Check sheet for the modelled part. Datum: model origin and axes. Units: mm. A direction names the side the tool comes from. Coordinates: 2 decimals unless noted, no trailing zeros. Write each loop counter-clockwise with the first axis right and the second up, starting at its lowest first coordinate (ties: lowest second). Pieces come first, ordered by that corner, then holes. Notation, with made-up numbers: (60.5, -1) -> (102.5, -1) arc R16 cw to (102.5, 15) -> close; hole circle Ø10 at (-39, -33). An arc over 180 degrees is marked (long way). One line per item, written item: value. Start each with the question number.
1) Draft check along Y on faces 1 (the flat face through (26, -22, 14)), 2 (the flat face through (-3.61, -1.36, 1.73)). Enter one of: +Y half, -Y half, draft (parallel to the pull), parting line (faces both ways), or undercut.
2) Gauge pin test, flat ends, axial feed: P1, Ø3, axis at x = -5.5, y = -0.5, coming from the -Z side; P2, Ø2.5, axis at x = -1, z = 9, coming from the -Y side; P3, Ø6, axis at x = 16, y = 30, coming from the +Z side. Record the tip position at first contact, or that the pin passes through.
3) Sectioned sample at A-A on x = 25. Enter the section's corners in (y, z), plus the area to 3 significant figures.
4) Scan lines: line 1 along Y through (x, z) = (-6, 5.5); line 2 along Y through (x, z) = (28, 9); line 3 along Y through (x, z) = (6, 10). Record each from-to range of solid material in increasing order. Write a range as [from, to].
5) Sectioned sample at D-D on z = 12.75. Give the number of separate pieces and of enclosed holes in the cut face, plus the area to 3 significant figures.
6) Set-up check for faces 3 (the flat face through (21, -32, 8)), 4 (the flat face through (-10, -1, 7)), 5 (the flat face through (8.37, -39.606, 1.726)), 6 (the cylindrical face through (-0.17, -41.3, 6.4)): record each of +Z, -Z, +X, -X, +Y, -Y from which the full face is reachable in a straight line by a thin tool's end or side.
7) Sectioned sample at B-B on y = -20. Enter the section's corners in (x, z), plus the area to 3 significant figures.
8) Sectioned sample at C-C on x = 0. Enter the section's corners in (y, z), plus the area to 3 significant figures.
```python
from build123d import *

# Parameters (mm, degrees)
PAD004_DEPTH    = 5
PAD003_DEPTH    = 5
PAD002_DEPTH    = 5
PAD001_DEPTH    = 5
SKETCH_W        = 45
SKETCH_H        = 90
PAD_DEPTH       = 14
SKETCH001_R     = 7.6
POCKET_DEPTH    = 90.001
SKETCH002_R     = 1.75
POCKET001_DEPTH = 14.001
POCKET002_DEPTH = 12
SKETCH004_R     = 2.25
POCKET003_DEPTH = 14.001
SKETCH008_R     = 4.1
POCKET005_DEPTH = 20
POCKET006_DEPTH = 3.5
POCKET007_DEPTH = 5


with BuildPart() as pad004:
    # Sketch021 → Pad004 (new body)
    with BuildSketch(Plane.XZ.offset(32.5)):
        with BuildLine():
            ThreePointArc((-7.6, 14), (0, 6.4), (7.6, 14))
            Line((7.6, 14), (5, 14))
            ThreePointArc((-5, 14), (0, 9), (5, 14))
            Line((-7.6, 14), (-5, 14))
        make_face()
    extrude(amount=PAD004_DEPTH)


with BuildPart() as pad003:
    # Sketch020 → Pad003 (new body)
    with BuildSketch(Plane.XZ.offset(-32.5)):
        with BuildLine():
            ThreePointArc((-7.6, 14), (0, 6.4), (7.6, 14))
            Line((7.6, 14), (5, 14))
            ThreePointArc((-5, 14), (0, 9), (5, 14))
            Line((-7.6, 14), (-5, 14))
        make_face()
    extrude(amount=-PAD003_DEPTH)


with BuildPart() as pad002:
    # Sketch019 → Pad002 (new body)
    with BuildSketch(Plane.XZ.offset(7.5)):
        with BuildLine():
            ThreePointArc((-7.6, 14), (0, 6.4), (7.6, 14))
            Line((7.6, 14), (5, 14))
            ThreePointArc((-5, 14), (0, 9), (5, 14))
            Line((-7.6, 14), (-5, 14))
        make_face()
    extrude(amount=-PAD002_DEPTH)


with BuildPart() as pad001:
    # Sketch018 → Pad001 (new body)
    with BuildSketch(Plane.XZ.offset(-7.5)):
        with BuildLine():
            ThreePointArc((-7.6, 14), (0, 6.4), (7.6, 14))
            Line((7.6, 14), (5, 14))
            ThreePointArc((-5, 14), (0, 9), (5, 14))
            Line((-7.6, 14), (-5, 14))
        make_face()
    extrude(amount=PAD001_DEPTH)


with BuildPart() as fusion:
    # Sketch → Pad (new body)
    with BuildSketch(Plane.XY):
        with Locations((12.5, 0)):
            Rectangle(SKETCH_W, SKETCH_H)
    extrude(amount=PAD_DEPTH)

    # Sketch001 → Pocket (cut, through all)
    with BuildSketch(Plane.XZ.offset(45)):
        with Locations((0, 14)):
            Circle(SKETCH001_R)
    extrude(amount=-POCKET_DEPTH, mode=Mode.SUBTRACT)

    # Sketch002 → Pocket001 (cut, through all)
    with BuildSketch(Plane.XY.offset(14)):
        with Locations((-6, 41)):
            Circle(SKETCH002_R)
        with Locations((-6, -41)):
            Circle(SKETCH002_R)
        with Locations((6, 41)):
            Circle(SKETCH002_R)
        with Locations((6, -41)):
            Circle(SKETCH002_R)
        with Locations((6, 0)):
            Circle(SKETCH002_R)
        with Locations((-6, 0)):
            Circle(SKETCH002_R)
        with Locations((28, 41)):
            Circle(SKETCH002_R)
        with Locations((28, 23)):
            Circle(SKETCH002_R)
        with Locations((28, -23)):
            Circle(SKETCH002_R)
        with Locations((28, -41)):
            Circle(SKETCH002_R)
    extrude(amount=-POCKET001_DEPTH, mode=Mode.SUBTRACT)

    # Sketch003 → Pocket002 (cut)
    with BuildSketch(Plane.XY.offset(14)):
        Polygon((10, 50), (10, -50), (21, -50), (21, -18), (41, -18), (41, 18), (21, 18), (21, 50), align=None)
    extrude(amount=-POCKET002_DEPTH, mode=Mode.SUBTRACT)

    # Sketch004 → Pocket003 (cut, through all)
    with BuildSketch(Plane(origin=(0, 0, 0), x_dir=(1, 0, 0), z_dir=(0, 0, -1))):
        with Locations((25, 7.5)):
            Circle(SKETCH004_R)
        with Locations((25, -7.5)):
            Circle(SKETCH004_R)
    extrude(amount=-POCKET003_DEPTH, mode=Mode.SUBTRACT)

    # Sketch008 → Pocket005 (cut)
    with BuildSketch(Plane.YZ.offset(35)):
        with Locations((-32.5, 14)):
            Circle(SKETCH008_R)
        with Locations((32.5, 14)):
            Circle(SKETCH008_R)
    extrude(amount=-POCKET005_DEPTH, mode=Mode.SUBTRACT)

    # Sketch012 → Pocket006 (cut)
    with BuildSketch(Plane(origin=(0, 0, 0), x_dir=(1, 0, 0), z_dir=(0, 0, -1))):
        Polygon((-4.412285, 2.750003), (-7.587715, 2.750003), (-9.17543, 0), (-7.587715, -2.750003), (-4.412285, -2.750003), (-2.82457, 0), align=None)
        Polygon((7.587715, 2.750003), (4.412285, 2.750003), (2.82457, 0), (4.412285, -2.750003), (7.587715, -2.750003), (9.17543, 0), align=None)
        Polygon((-4.412285, 43.750003), (-7.587715, 43.750003), (-9.17543, 41), (-7.587715, 38.249997), (-4.412285, 38.249997), (-2.82457, 41), align=None)
        Polygon((7.587715, -38.249997), (4.412285, -38.249997), (2.82457, -41), (4.412285, -43.750003), (7.587715, -43.750003), (9.17543, -41), align=None)
        Polygon((7.587715, 43.750003), (4.412285, 43.750003), (2.82457, 41), (4.412285, 38.249997), (7.587715, 38.249997), (9.17543, 41), align=None)
        Polygon((-4.412285, -38.249997), (-7.587715, -38.249997), (-9.17543, -41), (-7.587715, -43.750003), (-4.412285, -43.750003), (-2.82457, -41), align=None)
    extrude(amount=-POCKET006_DEPTH, mode=Mode.SUBTRACT)

    # Sketch022 → Pocket007 (cut)
    with BuildSketch(Plane.XY.offset(2)):
        Polygon((44.573685, 18), (36, 3.425), (36, -3.425), (44.573685, -18), (55.573685, -18), (55.573685, 18), align=None)
    extrude(amount=-POCKET007_DEPTH, mode=Mode.SUBTRACT)

    # Fusion: union Pad004, Pad003, Pad002, Pad001
    add(pad004.part)
    add(pad003.part)
    add(pad002.part)
    add(pad001.part)


solid = fusion.part
```
Answers:
1. face 1: draft
1. face 2: undercut
2. P1: stops at z = 3.5
2. P2: stops at y = -37.5
2. P3: stops at z = 2
3. outline: (-45, 0) -> (-9.75, 0) -> (-9.75, 2) -> (-18, 2) -> (-18, 14) -> (-28.4, 14) arc R4.1 cw to (-36.6, 14) -> (-45, 14) -> close; (-5.25, 0) -> (5.25, 0) -> (5.25, 2) -> (-5.25, 2) -> close; (9.75, 0) -> (45, 0) -> (45, 14) -> (36.6, 14) arc R4.1 cw to (28.4, 14) -> (18, 14) -> (18, 2) -> (9.75, 2) -> close
3. area: 757 mm2
4. line 1: y = [-45, -42.75], [-39.25, -1.75], [1.75, 39.25], [42.75, 45]
4. line 2: y = [-45, -42.75], [-39.25, -24.75], [-21.25, -18], [18, 21.25], [24.75, 39.25], [42.75, 45]
4. line 3: y = [-37.5, -32.5], [-7.5, -2.5], [2.5, 7.5], [32.5, 37.5]
5. separate pieces: 6
5. enclosed holes: 4
5. area: 1,050 mm2
6. face 3: +Z, +Y, -Y
6. face 4: +Z, -Z, -X, +Y, -Y
6. face 5: -Z
6. face 6: +Z, -Y
7. outline: (-10, 0) -> (35, 0) -> (35, 14) -> (21, 14) -> (21, 2) -> (10, 2) -> (10, 14) -> (7.6, 14) arc R7.6 cw to (-7.6, 14) -> (-10, 14) -> close
7. area: 407 mm2
8. outline: (-45, 0) -> (45, 0) -> (45, 6.4) -> (37.5, 6.4) -> (37.5, 9) -> (32.5, 9) -> (32.5, 6.4) -> (7.5, 6.4) -> (7.5, 9) -> (2.5, 9) -> (2.5, 6.4) -> (-2.5, 6.4) -> (-2.5, 9) -> (-7.5, 9) -> (-7.5, 6.4) -> (-32.5, 6.4) -> (-32.5, 9) -> (-37.5, 9) -> (-37.5, 6.4) -> (-45, 6.4) -> close
8. area: 628 mm2
